Model file for the job. Use its own axes, mm. Face numbers are marked on the shaded views. A direction names the side the tool comes from. Give positions to 0.01 mm unless a question says otherwise; leave off trailing zeros. Order: outer loops, then holes, each group sorted by start corner. A loop starts at its lowest first (then second) coordinate and runs counter-clockwise, first axis right, second up. Notation, with made-up numbers: (-1.75, -28.5) - (10.25, -28.5) arc R27 cw to (10.25, -6.5) - close; hole circle Ø5 at (85, 55). An arc over 180 degrees is marked (long way). Return JSON: item names as keys, results as strings. Group by question number.
from build123d import *

# Parameters (mm, degrees)
EXTRUDE_1_DEPTH          = 85
M4X0_7_1_D               = 3.3
M4X0_7_1_DEPTH           = 11.5
M4X0_7_1_TIP             = 0.991420021
M4X0_7_1_ON_FACE_2_D     = 3.3
M4X0_7_1_ON_FACE_2_DEPTH = 11.5
M4X0_7_1_ON_FACE_2_TIP   = 0.991420021


with BuildPart() as part:
    # ｽｹｯﾁ1 → ﾎﾞｽ - 押し出し1 (new body)
    with BuildSketch(Plane.XY):
        Polygon((0, 0), (0, 15), (2, 15), (2, 2), (15, 2), (15, 0), align=None)
    extrude(amount=EXTRUDE_1_DEPTH)

    # M4x0.7 ねじ穴1
    with Locations(Plane(origin=(0, 7.5, 75), x_dir=(0, 0, -1), z_dir=(-1, 0, 0))):
        with Locations((0, 0), (65, 0)):
            Hole(M4X0_7_1_D / 2, depth=M4X0_7_1_DEPTH)
            with Locations((0, 0, -(M4X0_7_1_DEPTH + M4X0_7_1_TIP / 2))):  # 118° drill point
                Cone(0, M4X0_7_1_D / 2, M4X0_7_1_TIP, mode=Mode.SUBTRACT)

    # M4x0.7 ねじ穴1 on face 2
    with Locations(Plane(origin=(7.5, 0, 75), x_dir=(0, 0, -1), z_dir=(0, -1, 0))):
        with Locations((0, 0), (65, 0)):
            Hole(M4X0_7_1_ON_FACE_2_D / 2, depth=M4X0_7_1_ON_FACE_2_DEPTH)
            with Locations((0, 0, -(M4X0_7_1_ON_FACE_2_DEPTH + M4X0_7_1_ON_FACE_2_TIP / 2))):  # 118° drill point
                Cone(0, M4X0_7_1_ON_FACE_2_D / 2, M4X0_7_1_ON_FACE_2_TIP, mode=Mode.SUBTRACT)


solid = part.part
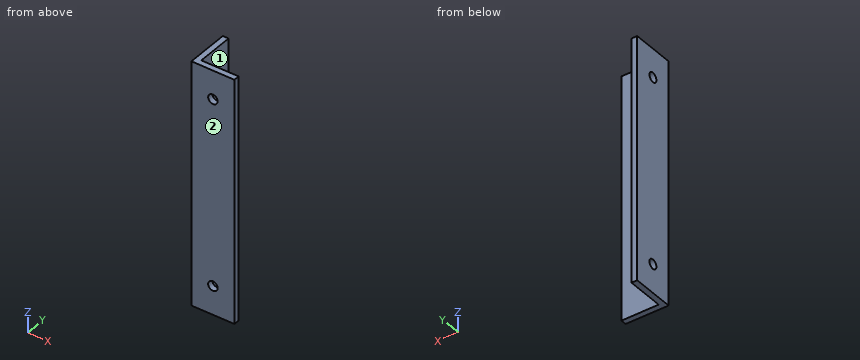
(1) Slice it at A-A (z = 75). Give the cut face in (x, y), and give its area (3 significant figures).
(2) Slice it at D-D (z = 65.5). Give the cut face in (x, y), and give its area (3 significant figures).
(3) 3-axis set-ups, long thin cutter, end or side, ignore diameter. For the marked faces 1 and 2: which of +Z, -Z, +X, -X, +Y, -Y reach the whole face in a straight line?
(4) Slice it at B-B (y = 7.5). Give the cut face in (x, z).
(5) Drill centre lines: L1, parallel to Y at x = 0.9, z = 10; L2, parallel to Y at x = 6.5, z = 43.5. Where is each one in solid material? Low to high.
(6) Drop flat-ended pins along their axis: pin 1 Ø4 at (y, z) = (6.5, 43.5) entering from +X; pin 2 Ø4 at (x, z) = (10.5, 57) entering from +Y. Give the stop position or say it passes through.
Result set:
{
 "1": {"outline": "(0, 0) - (5.85, 0) - (5.85, 2) - (2, 2) - (2, 5.85) - (0, 5.85) - close; (0, 9.15) - (2, 9.15) - (2, 15) - (0, 15) - close; (9.15, 0) - (15, 0) - (15, 2) - (9.15, 2) - close", "area": "42.8 mm²"},
 "2": {"outline": "(0, 0) - (15, 0) - (15, 2) - (2, 2) - (2, 15) - (0, 15) - close", "area": "56.0 mm²"},
 "3": {"face 1": "+Z, -Z, +X, +Y", "face 2": "+Z, -Z, +X, -X, -Y"},
 "4": {"outline": "(0, 0) - (2, 0) - (2, 8.35) - (0, 8.35) - close; (0, 11.65) - (2, 11.65) - (2, 73.35) - (0, 73.35) - close; (0, 76.65) - (2, 76.65) - (2, 85) - (0, 85) - close"},
 "5": {"L1": "y = 0 to 5.85, 9.15 to 15", "L2": "y = 0 to 2"},
 "6": {"pin 1": "stops at x = 2", "pin 2": "stops at y = 2"}
}
